Work out the finished part from the listing and answer in its coordinate system (mm). A direction names the side the tool comes from. Coordinates: 2 decimals unless noted, no trailing zeros. Write each loop counter-clockwise with the first axis right and the second up, starting at its lowest first coordinate (ties: lowest second). Pieces come first, ordered by that corner, then holes. Notation, with made-up numbers: (-5, 26.25) - (10, 26.25) arc R29 ccw to (10, 62.25) - close; hole circle Ø4 at (25, 89.25). An arc over 180 degrees is marked (long way). Use a Markdown table: item, result. Add a question column.
(1) Find the intervals of material crossed by line 1 (Z direction, x = 0, y = -9.75); line 2 (Z direction, x = 0.5, y = -14.5); line 3 (X direction, y = -13, z = 12.5), in increasing order. Write a range as from..to.
(2) A tool of negligible diameter and unlimited length cuts with its end or side. For faces 4 (the face through (0.54, -7.6, -10.06)), 5 (the face through (0, -28, 18)), from which of +Z, -Z, +X, -X, +Y, -Y can it reach the whole face along a straight path? Write none if from no direction.
(3) For a pull along Z with two mould halves and no side action, classify faces 1 (the face through (0, 0, 0)), 2 (the face through (0.23, -16.24, 12.13)), 3 (the face through (0, -28, -18)) as released by +Z, released by -Z, zero draft, split by the parting line, or undercut.
(4) The part is cut by section A-A, the plane y = -5. Give the vertices of the cut face in (x, z).
(5) Given pin 1 Ø1.5 at (x, z) = (3, 13) entering from +Y; pin 2 Ø3 at (x, z) = (0, 12.5) entering from +Y, each flat-ended and moving along its own axis, determine where each tip first touches the part or whether it passes through.
from build123d import *

# Parameters (mm, degrees)
SKETCH1_W             = 15
SKETCH1_H             = 36
BOSS_EXTRUDE1_DEPTH   = 57
M6_TAPPED_HOLE1_D     = 5
M6_TAPPED_HOLE1_DEPTH = 15
M6_TAPPED_HOLE1_TIP   = 1.502151548


with BuildPart() as part:
    # Sketch1 → Boss-Extrude1 (new body)
    with BuildSketch(Plane(origin=(0, 0, 0), x_dir=(1, 0, 0), z_dir=(0, 1, 0))):
        Rectangle(SKETCH1_W, SKETCH1_H)
    extrude(amount=-BOSS_EXTRUDE1_DEPTH)

    # M6 Tapped Hole1
    with Locations(Plane(origin=(0, 0, 0), x_dir=(1, 0, 0), z_dir=(0, 1, 0))):
        with Locations((0, 12.5), (0, -12.5)):
            Hole(M6_TAPPED_HOLE1_D / 2, depth=M6_TAPPED_HOLE1_DEPTH)
            with Locations((0, 0, -(M6_TAPPED_HOLE1_DEPTH + M6_TAPPED_HOLE1_TIP / 2))):  # 118° drill point
                Cone(0, M6_TAPPED_HOLE1_D / 2, M6_TAPPED_HOLE1_TIP, mode=Mode.SUBTRACT)


solid = part.part
Model answer:
| question | item | result |
|---|---|---|
| 1 | line 1 | -18..-15, -10..10, 15..18 |
| 1 | line 2 | -18..-14.95, -10.05..10.05, 14.95..18 |
| 1 | line 3 | -7.5..-2.5, 2.5..7.5 |
| 2 | face 4 | +Y |
| 2 | face 5 | +Z, +X, -X, +Y, -Y |
| 3 | face 1 | zero draft |
| 3 | face 2 | undercut |
| 3 | face 3 | released by -Z |
| 4 | outline | (-7.5, -18) - (7.5, -18) - (7.5, 18) - (-7.5, 18) - close; hole circle Ø5 at (0, -12.5); hole circle Ø5 at (0, 12.5) |
| 5 | pin 1 | y = 0 |
| 5 | pin 2 | y = -15.6 |
